Model file for the job. Use its own axes, mm. A direction names the side the tool comes from. Round coordinates to 2 decimals unless told otherwise and drop trailing zeros. Order: outer loops, then holes, each group sorted by start corner. A loop starts at its lowest first (then second) coordinate and runs counter-clockwise, first axis right, second up. Notation, with made-up numbers: (-11, -22) -> (30, -22) arc R3 ccw to (30, -17) -> close; hole circle Ø7 at (57, 25). An arc over 180 degrees is marked (long way). Put each result on its own line as item: value. Start each with the question number.
Q1. Cut at A-A, the plane z = 9.25. List the corners of the cut face in (x, y).
Q2. Probe L1, parallel to Z at x = 3.75, y = 15.75 (3 decimals); L2, parallel to X at y = 17.25, z = 3.75 (3 decimals); L3, parallel to Y at x = 1.75, z = 8. List the from-to ranges inside material, lowest first.
Q3. Cut at C-C, the plane x = 7. List the corners of the cut face in (y, z), and give its area (3 significant figures).
Q4. 3-axis set-ups, long thin cutter, end or side, ignore diameter. For faces 1 (the face through (0, 13, -2.5)), 2 (the face through (-8, -4.75, 5)), 3 (the face through (6.25, 0, 5)), 4 (the face through (7, 0, 0)): which of +Z, -Z, +X, -X, +Y, -Y reach the whole face in a straight line?
Q5. Pull direction Y, two halves, no side cores. Call faces 5 (the face through (0, -9.75, 4)), 6 (the face through (0, 7.25, 5)), 7 (the face through (-8.75, 12, 4)): released by +Y, released by -Y, zero draft, split by the parting line, or undercut.
Q6. Cut at B-B, the plane y = -6.75. List the corners of the cut face in (x, z), and give its area (4 significant figures).
Q7. Flat gauge pins, fed straight in: P1, Ø3, axis at x = 7.5, y = -2.5, coming from the -Z side; P2, Ø3, axis at x = 3.75, z = 3.75, coming from the +Y side; P3, Ø6, axis at x = -6.5, y = -6, coming from the -Z side. Where does each tip first touch, or does it go through?
Autodesk Inventor part; units mm, degrees
ref_plane "YZ Plane" through (0, 0, 0) normal (1, 0, 0) x (0, 1, 0)
ref_plane "XZ Plane" through (0, 0, 0) normal (0, 1, 0) x (-1, 0, 0)
ref_plane "XY Plane" through (0, 0, 0) normal (0, 0, 1) x (1, 0, 0)
sketch "Sketch1" plane through (0, 0, 0) normal (0, 0, 1) x (1, 0, 0)
  line L0 (-6.25, -7.25) -> (6.25, -7.25)
  line L1 (6.25, -7.25) -> (6.25, 7.25)
  line L2 (6.25, 7.25) -> (-6.25, 7.25)
  line L3 (-6.25, 7.25) -> (-6.25, -7.25)
  line L4 (-6.25, -7.25) -> (6.25, 7.25) construction
  line L5 (6.25, -7.25) -> (-6.25, 7.25) construction
  line L6 (-8.75, -9.75) -> (8.75, -9.75)
  line L7 (8.75, -9.75) -> (8.75, 9.75)
  line L8 (8.75, 9.75) -> (-8.75, 9.75)
  line L9 (-8.75, 9.75) -> (-8.75, -9.75)
  line L10 (-8.75, -9.75) -> (8.75, 9.75) construction
  line L11 (8.75, -9.75) -> (-8.75, 9.75) construction
  point P0 (0, 0)
  dimension "d0" = 12.5
  dimension "d1" = 14.5
  dimension "d2" = 17.5
  dimension "d3" = 19.5
extrude "Extrusion1" add sketch "Sketch1" along normal blind 10
sketch "Sketch2" plane through (0, 0, 0) normal (0, 0, -1) x (-1, 0, 0)
  line L0 (8.75, 9.75) -> (8.75, -9.75)
  line L1 (-8.75, 9.75) -> (8.75, 9.75)
  line L2 (8.75, 9.75) -> (8.75, 6.25)
  line L3 (8.75, 6.25) -> (-8.75, 6.25)
  line L4 (-8.75, 6.25) -> (-8.75, 9.75)
  line L5 (6.25, 7.25) -> (-6.25, 7.25)
  line L6 (-8.75, -9.75) -> (-8.75, 9.75)
  line L7 (-8.75, -9.75) -> (8.75, -9.75)
  line L8 (8.75, -9.75) -> (8.75, -6.25)
  line L9 (8.75, -6.25) -> (-8.75, -6.25)
  line L10 (-8.75, -6.25) -> (-8.75, -9.75)
  line L11 (-6.25, -7.25) -> (6.25, -7.25)
  point P0 (0, 0)
  point P1 (-8.75, -6.25)
  dimension "d6" = 1
  dimension "d7" = 1
extrude "Extrusion2" add sketch "Sketch2" along normal blind 2.5 contours L0 L3 L4 L1 | L0 L7 L6 L9
thicken "Thicken1" operation add thickness 10.199 both sides no extend neighbours no toward (0, 1, 0) faces at (-2.9167, 9.75, 5.8333)
sketch "Sketch3" plane through (-8.75, 19.949, 10) normal (0, 1, 0) x (1, 0, 0)
  line L0 (0, 12.5) -> (0, 0)
  line L1 (17.5, 12.5) -> (17.5, 0)
  point P0 (8.75, 10)
  point P1 (12.5, 6.25)
  point P2 (0, 6.25)
  dimension "d19" = 5
hole "Hole1" at (3.75, 19.949, 3.75) direction (0, -1, 0) diameter 5.35 depth 10 tip angle 118
sketch "Sketch4" plane through (-8.75, -6.25, 0) normal (-1, 0, 0) x (0, 0, 1)
  line L0 (10, -3.5) -> (10, 26.199)
  line L1 (0, 12.5) -> (0, 0)
  line L2 (10, 1.5) -> (0, 1.5)
  line L3 (0, 1.5) -> (0, 11)
  line L4 (0, 11) -> (10, 11)
  line L5 (10, 11) -> (10, 1.5)
  line L6 (-2.5, -3.5) -> (10, -3.5)
  point P0 (0, 6.25)
  point P1 (0, 1.5)
  dimension "d20" = 5
  dimension "d21" = 9.5
extrude "Extrusion3" cut sketch "Sketch4" against normal blind 5
properties part number "Adafruit_1528_4663-ND_House_02"
Ans:
1. outline: (-8.75, -9.75) -> (8.75, -9.75) -> (8.75, 19.95) -> (-8.75, 19.95) -> (-8.75, 4.75) -> (-6.25, 4.75) -> (-6.25, 7.25) -> (6.25, 7.25) -> (6.25, -7.25) -> (-6.25, -7.25) -> (-6.25, -4.75) -> (-8.75, -4.75) -> close
2. L1: z = -2.5 to 1.075, 6.425 to 10
2. L2: x = -8.75 to 1.075, 6.425 to 8.75
2. L3: y = -9.75 to -7.25, 7.25 to 19.95
3. outline: (-9.75, -2.5) -> (-6.25, -2.5) -> (-6.25, 0) -> (6.25, 0) -> (6.25, -2.5) -> (19.95, -2.5) -> (19.95, 10) -> (-9.75, 10) -> close
3. area: 340 mm^2
4. face 1: -Z, +X, -X, +Y, -Y
4. face 2: +Z, -Z, -X
4. face 3: +Z
4. face 4: -Z, +X, -X
5. face 5: released by -Y
5. face 6: undercut
5. face 7: zero draft
6. outline: (-8.75, -2.5) -> (8.75, -2.5) -> (8.75, 10) -> (6.25, 10) -> (6.25, 0) -> (-6.25, 0) -> (-6.25, 10) -> (-8.75, 10) -> close
6. area: 93.75 mm^2
7. P1: stops at z = 0
7. P2: stops at y = 9.24
7. P3: stops at z = -2.5
